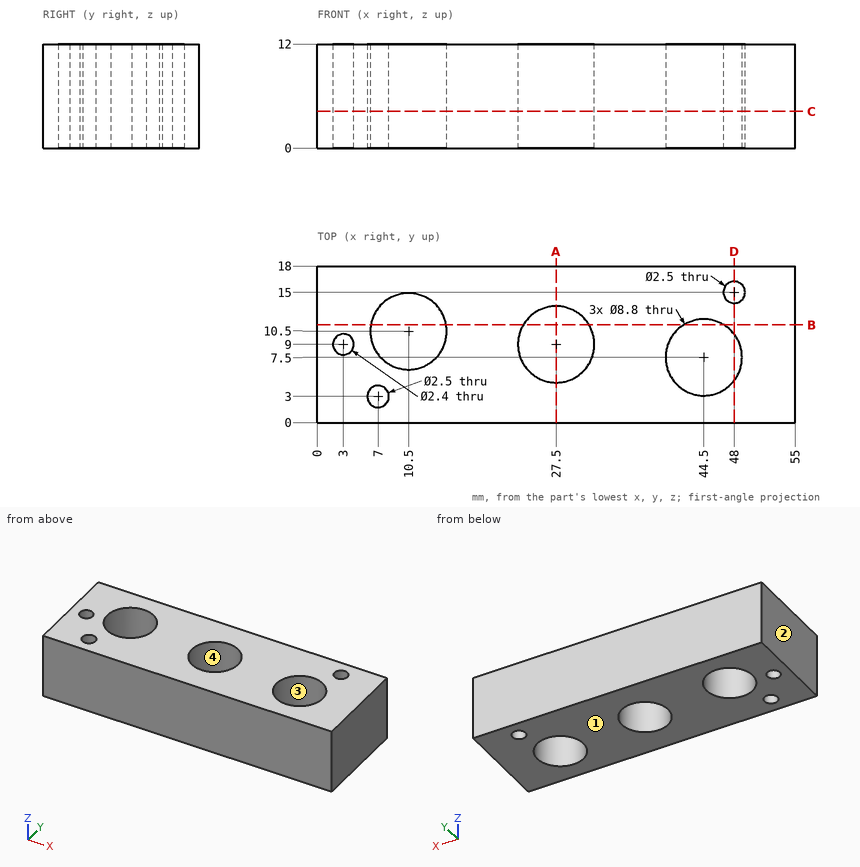
Could you check a few things on this drawing? It's one solid part, dimensions in mm from its lowest x, y, z. Coordinates: 2 decimals unless noted, no trailing zeros. Write each loop counter-clockwise with the first axis right and the second up, starting at its lowest first coordinate (ties: lowest second). Pieces come first, ordered by that corner, then holes.
Q1. Please list where these lines run through material, in increasing order: L1, parallel to Y at x = 3, z = 3.25; L2, parallel to Y at x = 10.5, z = 8; L3, parallel to X at y = 9.25, z = 3.5.
Results found:
L1: y = 0 to 7.8, 10.2 to 18
L2: y = 0 to 6.1, 14.9 to 18
L3: x = 0 to 1.83, 4.17 to 6.28, 14.72 to 23.11, 31.89 to 40.46, 48.54 to 55
Q2. Imagine slicing it at C-C, the plane z = 4.25. List the corners of the cut face in (x, y) for me.
Results found:
outline: (0, 0) - (55, 0) - (55, 18) - (0, 18) - close; hole circle Ø2.4 at (3, 9); hole circle Ø2.5 at (7, 3); hole circle Ø8.8 at (10.5, 10.5); hole circle Ø8.8 at (27.5, 9); hole circle Ø8.8 at (44.5, 7.5); hole circle Ø2.5 at (48, 15)
Q3. Imagine slicing it at D-D, the plane x = 48. List the corners of the cut face in (y, z) for me.
Results found:
outline: (0, 0) - (4.83, 0) - (4.83, 12) - (0, 12) - close; (10.17, 0) - (13.75, 0) - (13.75, 12) - (10.17, 12) - close; (16.25, 0) - (18, 0) - (18, 12) - (16.25, 12) - close
Q4. If we mould it in two halves opening along X, with no side actions, what happens to the marked faces 1, 2, 3 and 4? For each: +X half, -X half, draft (parallel to the pull), parting line (faces both ways), or undercut.
Results found:
face 1: draft
face 2: -X half
face 3: undercut
face 4: undercut
Q5. Imagine slicing it at B-B, the plane y = 11.25. List the corners of the cut face in (x, z) for me, plus the area to 3 significant figures.
Results found:
outline: (0, 0) - (6.16, 0) - (6.16, 12) - (0, 12) - close; (14.84, 0) - (23.72, 0) - (23.72, 12) - (14.84, 12) - close; (31.28, 0) - (42.2, 0) - (42.2, 12) - (31.28, 12) - close; (46.8, 0) - (55, 0) - (55, 12) - (46.8, 12) - close
area: 410 mm2
Q6. Imagine slicing it at A-A, the plane x = 27.5. List the corners of the cut face in (y, z) for me.
Results found:
outline: (0, 0) - (4.6, 0) - (4.6, 12) - (0, 12) - close; (13.4, 0) - (18, 0) - (18, 12) - (13.4, 12) - close
Q7. For P1, Ø5, axis at x = 36, y = 7.5, coming from the -Z side, with a flat end and sliding along its axis, tell me the tip position at first contact or that it passes through.
Results found:
P1: stops at z = 0
